Model file for the job. Use its own axes, mm. A direction names the side the tool comes from. Coordinates: 2 decimals unless noted, no trailing zeros. Loops run counter-clockwise (first coordinate to the right, second up) from the corner with the lowest first, then second, coordinate; pieces in that order, holes last. Notation, with made-up numbers: M -4,59.5 L 45,59.5 A20 ccw 45,86.5 Z; hole C 23,62 d2. An arc over 180 degrees is marked long. One line per question, with ' | ' between items. Start each with the question number.
Autodesk Inventor part; units mm, degrees
ref_plane "Work Plane1" through (0, 0, 12.7) normal (0, 0, 1) x (1, 0, 0)
ref_plane "YZ Plane" through (0, 0, 0) normal (1, 0, 0) x (0, 1, 0)
ref_plane "XZ Plane" through (0, 0, 0) normal (0, 1, 0) x (-1, 0, 0)
sketch "Sketch1" plane through (0, 0, 0) normal (0, 0, 1) x (1, 0, 0)
  line L0 (46.95, 0) -> (46.95, 38.1)
  line L1 (46.95, 38.1) -> (59.65, 38.1)
  line L2 (59.65, 38.1) -> (72.35, 38.1)
  line L3 (72.35, 38.1) -> (72.35, 0)
  circle A0 centre (61.35, -6.35) radius 12.065
  line L4 (46.95, 38.1) -> (47.2, 38.1)
  line L5 (47.2, 38.1) -> (47.2, 37.85)
  line L6 (72.35, 0) -> (72.1, 0)
  line L7 (72.1, 0) -> (72.1, 0.25)
  line L8 (72.1, 0.25) -> (47.2, 0.25)
  line L9 (47.2, 0.25) -> (47.2, 37.85)
  line L10 (47.2, 37.85) -> (72.1, 37.85)
  line L11 (72.1, 37.85) -> (72.1, 0.25)
  point P0 (0, 0)
  dimension "d0" = 0.25
  dimension "d1" = 0.25
  dimension "d2" = 0.25
  dimension "d3" = 0.25
extrude "Extrusion1" add sketch "Sketch1" against normal blind 5 contours L10 L11 L8 A0 L9 | A0 L8 picked at (62.9802, 2.7077)
sketch "Sketch2" plane through (0, 0, 0) normal (0, 0, 1) x (1, 0, 0)
  line L0 (47.2, 37.85) -> (72.1, 37.85)
  line L1 (47.2, 37.85) -> (47.2, 12.958)
  line L2 (72.1, 37.85) -> (72.1, 0.25)
  circle A0 centre (59.6397, 25.404) radius 12.446
  line L3 (47.2, 0.25) -> (47.2, 37.85)
  line L4 (47.2, 25.7997) -> (72.1, 25.7997)
  line L5 (72.1, 25.7997) -> (72.1, 0.25)
  line L6 (72.1, 0.25) -> (47.2, 0.25)
  line L7 (47.2, 0.25) -> (47.2, 25.7997)
  point P0 (0, 0)
  dimension "d6" = 24.892
extrude "Extrusion2" add sketch "Sketch2" along normal blind 25.4 contours A0 L4 | L4 A0 L1 | L1 A0 | L4 L2 L6 L3 L1 A0
sketch "Sketch3" plane through (0, 0, 25.4) normal (0, 0, 1) x (1, 0, 0)
  circle A0 centre (61.35, -6.35) radius 12.065
  circle A1 centre (61.35, -6.35) radius 6.35
  line L0 (72.1, 37.85) -> (72.1, 0.25)
  line L1 (72.1, 0.25) -> (14.95, 0.25)
  line L2 (14.95, 0.25) -> (14.95, -14.99)
  line L3 (14.95, -14.99) -> (72.1, -14.99)
  line L4 (72.1, -14.99) -> (72.1, 0.25)
  line L5 (14.95, 0.25) -> (72.1, 0.25)
  line L6 (72.1, 0.25) -> (72.1, 10.41)
  point P0 (0, 0)
  dimension "d9" = 15.24
  dimension "d10" = 57.15
extrude "Extrusion3" add sketch "Sketch3" against normal blind 25.4 contours L4 A0 L3 L1 | A0 L1 L4 | L4 L3 A0 | A0 L3 L2 L1 | A1
sketch "Sketch5" plane through (72.1, -14.99, 0) normal (0, -1, 0) x (1, 0, 0)
  line L0 (-57.15, 25.4) -> (-57.15, 0)
  line L1 (-65.6167, 4.2333) -> (-57.15, 0)
  line L2 (-65.6167, 4.2333) -> (-57.15, 8.4667)
  line L3 (-65.6167, 21.1667) -> (-57.15, 25.4)
  line L4 (-65.6167, 21.1667) -> (-57.15, 16.9333)
  line L5 (-57.15, 16.9333) -> (-65.6167, 12.7)
  line L6 (-65.6167, 12.7) -> (-57.15, 8.4667)
  line L7 (0, 25.4) -> (0, 0)
  line L8 (-57.15, 25.4) -> (0, 25.4)
  line L9 (0, 25.4) -> (0, 0)
  line L10 (0, 0) -> (-57.15, 0)
  line L11 (0, 0) -> (-57.15, 0)
  line L12 (-57.15, 0) -> (-65.6167, 4.2333)
  line L13 (-65.6167, 4.2333) -> (-57.15, 8.4667)
  line L14 (-57.15, 8.4667) -> (-65.6167, 12.7)
  line L15 (-65.6167, 12.7) -> (-57.15, 16.9333)
  line L16 (-57.15, 16.9333) -> (-65.6167, 21.1667)
  line L17 (-65.6167, 21.1667) -> (-57.15, 25.4)
  point P0 (-72.1, 0)
  dimension "d16" = 8.4667
extrude "Extrusion5" add sketch "Sketch5" against normal blind 5.08
sketch "Sketch6" plane through (0, 0, 25.4) normal (0, 0, 1) x (1, 0, 0)
  line L0 (14.95, 0.25) -> (14.95, -9.91)
  line L1 (14.95, -9.91) -> (14.95, 0.25)
  line L2 (14.95, 0.25) -> (47.2, 0.25)
  arc A0 (47.2, 0.25) -> (14.95, -9.91) centre (44.4515, -47.2897) ccw
  point P0 (0, 0)
  point P1 (41.7029, 0.25)
extrude "Extrusion6" cut sketch "Sketch6" against normal blind 2540 contours L2 A0 L0
ref_plane "Work Plane1" through (0, 0, 12.7) normal (0, 0, 1) x (1, 0, 0)
sketch "Sketch7" plane through (0, 0, 12.7) normal (0, 0, 1) x (1, 0, 0)
  circle A0 centre (61.4402, -11.9143) radius 6.5
  line L0 (61.4402, -5.4143) -> (61.4402, -4.4143)
  line L1 (61.4402, -4.4143) -> (54.9402, -4.4143)
  line L2 (54.9402, -4.4143) -> (53.9402, -4.4143)
  line L3 (53.9402, -4.4143) -> (53.9402, -14.99)
  line L4 (14.95, -14.99) -> (72.1, -14.99)
  line L5 (53.9402, -14.99) -> (67.9402, -14.99)
  line L6 (67.9402, -14.99) -> (68.9402, -14.99)
  line L7 (68.9402, -14.99) -> (68.9402, -4.4143)
  line L8 (68.9402, -4.4143) -> (53.9402, -4.4143)
  line L9 (53.9402, -4.4143) -> (68.9402, -4.4143)
  line L10 (68.9402, -4.4143) -> (68.9402, -14.99)
  line L11 (68.9402, -14.99) -> (53.9402, -14.99)
  line L12 (53.9402, -14.99) -> (53.9402, -4.4143)
  point P0 (0, 0)
  dimension "d27" = 1
  dimension "d28" = 1
  dimension "d29" = 1
extrude "Extrusion7" cut sketch "Sketch7" along normal mid plane 6 contours A0 L4 | A0 L0 L8 L7 L4 | A0 L4 L3 L2 L1 L0 picked at (61.4402, -11.7981)
sketch "Sketch8" plane through (0, 0, 0) normal (0, 0, -1) x (-1, 0, 0)
  circle A0 centre (-61.4402, -11.9143) radius 2
  circle A1 centre (-61.4402, -11.9143) radius 1.75
  point P0 (0, 0)
  dimension "d34" = 3.5
extrude "Extrusion8" cut sketch "Sketch8" against normal blind 12.7 contours A1
sketch "Sketch9" plane through (0, 0, 0) normal (0, 0, -1) x (-1, 0, 0)
  line L0 (-53.9402, -14.99) -> (-68.9402, -14.99)
  line L1 (-61.4402, -14.99) -> (-66.4402, -14.99)
  line L2 (-61.4402, -14.99) -> (-56.4402, -14.99)
  line L3 (-56.4402, -14.99) -> (-56.4402, -10.1643)
  circle A0 centre (-61.4402, -11.9143) radius 1.75
  line L4 (-56.4402, -11.9143) -> (-56.4402, -8.8385)
  line L5 (-56.4402, -8.8385) -> (-66.4402, -8.8385)
  line L6 (-66.4402, -8.8385) -> (-66.4402, -14.99)
  point P0 (0, 0)
  dimension "d35" = 5
  dimension "d36" = 5
  dimension "d37" = 3.0757
  dimension "d38" = 3.0757
extrude "Extrusion9" cut sketch "Sketch9" against normal blind 5
sketch "Sketch10" plane through (0, 0, 15.7) normal (0, 0, -1) x (-1, 0, 0)
  circle A0 centre (-61.4402, -11.9143) radius 2
  circle A1 centre (-61.4402, -11.9143) radius 1.75
  point P0 (0, 0)
extrude "Extrusion10" cut sketch "Sketch10" against normal blind 5 contours A1
fillet "Fillet1" radius 0.5 3 edges at (6.4833, -12.45, 4.2333) (6.4833, -12.45, 12.7) (6.4833, -12.45, 21.1667)
sketch "Sketch11" plane through (0, 0, -5) normal (0, 0, -1) x (-1, 0, 0)
  line L0 (-72.1, 37.85) -> (-72.1, 0.25)
  line L1 (-47.2, 0.25) -> (-47.2, 37.85)
  line L2 (-72.1, 37.85) -> (-47.2, 37.85)
  line L3 (-47.2, 37.85) -> (-47.2, 25.15)
  line L4 (-47.2, 25.15) -> (-72.1, 25.15)
  line L5 (-72.1, 25.15) -> (-72.1, 37.85)
  point P0 (0, 0)
  dimension "d44" = 12.7
extrude "Extrusion11" cut sketch "Sketch11" against normal blind 5.08
equation "\"d38\" = d37"
properties part number "Leg"
(1) Band-saw the part on C-C on y = -6. Write the cut outline in (x, z).
(2) Band-saw the part on D-D on x = 45. Write the cut outline in (y, z).
(3) Pin check, flat tips, straight feed: P1, Ø1.8, axis at x = 60.5, z = 13.5, coming from the -Y side; P2, Ø3, axis at x = 15.5, z = 17.5, coming from the +Y side; P3, Ø4, axis at x = 10.5, z = 20.5, coming from the +Y side; P4, Ø12, axis at x = 30.5, y = 9.5, coming from the +Z side (3 decimals). Stop position of each tip, or through.
(4) Band-saw the part on A-A on x = 61. Write the cut outline in (y, z).
(5) Two-plate mould, pull along X, no slides. Class faces 1 (the face through (61, -10, 15.7)), 2 (the face through (47.2, 13, 10)), 3 (the face through (60, 30, 0.08)): pulls with the +X half, pulls with the -X half, needs draft (parallel to the pull), parting line crosses it, or undercut.
(6) 3-axis set-ups, long thin cutter, end or side, ignore diameter. For faces 4 (the face through (11.111, -12.486, 6.547)), 5 (the face through (60, 0.25, -2)), 6 (the face through (61, -10, 9.7)), 7 (the face through (44, 0.25, 13)): which of +Z, -Z, +X, -X, +Y, -Y reach the whole face in a straight line?
(7) Drill centre lines: line 1 (Z direction, x = 54.5, y = -4.5); line 2 (X direction, y = 12, z = 12); line 3 (Y direction, x = 65, z = -1). Where is each one in solid material? Low to high. Write a range as [from, to].
Computed values:
1) outline: M 20.73,0 L 72.1,0 L 72.1,25.4 L 20.73,25.4 Z; hole M 53.94,9.7 L 68.94,9.7 L 68.94,15.7 L 53.94,15.7 Z
2) outline: M -14.99,0 L 0.25,0 L 0.25,25.4 L -14.99,25.4 Z
3) P1: y = -4.41 | P2: y = -8.38 | P3: y = -9.91 | P4: through
4) outline: M -14.99,5 L -13.61,5 L -13.61,9.7 L -14.99,9.7 Z; M -14.99,15.7 L -13.61,15.7 L -13.61,20.7 L -10.22,20.7 L -10.22,15.7 L -4.41,15.7 L -4.41,9.7 L -10.22,9.7 L -10.22,5 L -8.84,5 L -8.84,0 L 0.25,0 L 0.25,-5 L 25.15,-5 L 25.15,0.08 L 37.78,0.08 L 37.78,25.4 L -14.99,25.4 Z
5) face 1: undercut | face 2: pulls with the -X half | face 3: needs draft
6) face 4: -X, +Y, -Y | face 5: -Z, +X, -X, -Y | face 6: -Y | face 7: +Z, -Z, -X, +Y
7) line 1: [0, 9.7], [15.7, 25.4] | line 2: [47.2, 72.1] | line 3: [0.25, 25.15]
